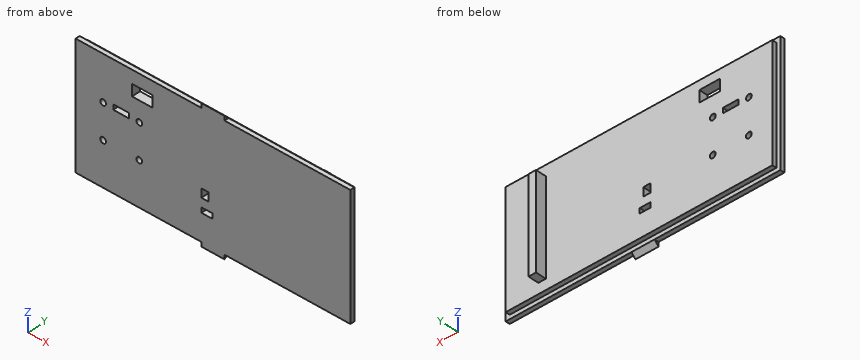
```python
from build123d import *

# Parameters (mm, degrees)
SKETCH2_W               = 190
SKETCH2_H               = 85
BOSS_EXTRUDE1_DEPTH     = 3
SKETCH6_W               = 184.4
SKETCH6_H               = 79.4
BOSS_EXTRUDE4_DEPTH     = 3
SKETCH8_W               = 16
SKETCH8_H               = 3
BOSS_EXTRUDE5_DEPTH     = 3
CHAMFER2_SIZE           = 3
CUT_EXTRUDE1_DEPTH      = 210.475535564
CUT_EXTRUDE1_DEPTH_BACK = 210.475535564
SKETCH10_W              = 7.5
SKETCH10_H              = 3.5
SKETCH11_W              = 5
SKETCH11_H              = 6
CUT_EXTRUDE2_DEPTH      = 210.475535564
SKETCH12_R              = 2
SKETCH12_W              = 11
SKETCH12_H              = 3.5
CUT_EXTRUDE3_DEPTH      = 210.475535564
SKETCH13_W              = 14.2
SKETCH13_H              = 8
CUT_EXTRUDE4_DEPTH      = 210.475535564
SKETCH14_W              = 5.173747918
SKETCH14_H              = 65
BOSS_EXTRUDE6_DEPTH     = 7.3


with BuildPart() as part:
    # Sketch2 → Boss-Extrude1 (new body)
    with BuildSketch(Plane(origin=(0, 0, 0), x_dir=(1, 0, 0), z_dir=(0, 1, 0))):
        with Locations((-95, 42.5)):
            Rectangle(SKETCH2_W, SKETCH2_H)
    extrude(amount=BOSS_EXTRUDE1_DEPTH)

    # Sketch6 → Boss-Extrude4 (add)
    with BuildSketch(Plane(origin=(0, 3, 0), x_dir=(1, 0, 0), z_dir=(0, 1, 0))):
        with Locations((-95, 42.5)):
            Rectangle(SKETCH6_W, SKETCH6_H)
    extrude(amount=BOSS_EXTRUDE4_DEPTH)

    # Sketch8 → Boss-Extrude5 (add)
    with BuildSketch(Plane(origin=(0, 3, 0), x_dir=(1, 0, 0), z_dir=(0, 1, 0))):
        with Locations((-95, -1.5)):
            Rectangle(SKETCH8_W, SKETCH8_H)
        with Locations((-95, 86.5)):
            Rectangle(SKETCH8_W, SKETCH8_H)
    extrude(amount=-BOSS_EXTRUDE5_DEPTH)

    # Chamfer2
    chamfer2_edges = [part.edges().sort_by_distance(p)[0] for p in [
        (-95, 3, 3),
        (-95, 3, -88),
    ]]
    chamfer(chamfer2_edges, length=CHAMFER2_SIZE - 0.0001)  # a hair under: the kernel refuses the full size

    # Sketch10 → Cut-Extrude1 (cut, two sides: drawn at the far end of the back side and taken through both)
    with BuildSketch(Plane.XZ.offset(-CUT_EXTRUDE1_DEPTH_BACK)):
        with Locations((-99.25, -64.75)):
            Rectangle(SKETCH10_W, SKETCH10_H)
    extrude(amount=CUT_EXTRUDE1_DEPTH + CUT_EXTRUDE1_DEPTH_BACK, mode=Mode.SUBTRACT)

    # Sketch11 → Cut-Extrude2 (cut, through all)
    with BuildSketch(Plane.XZ):
        with Locations((-100.5, -54)):
            Rectangle(SKETCH11_W, SKETCH11_H)
    extrude(amount=-CUT_EXTRUDE2_DEPTH, mode=Mode.SUBTRACT)

    # Sketch12 → Cut-Extrude3 (cut, through all)
    with BuildSketch(Plane.XZ):
        with Locations(Location((-171, -54.875455527, 0), (0, 0, 270))):
            Circle(SKETCH12_R)
        with Locations(Location((-171, -30.875455527, 0), (0, 0, 270))):
            Circle(SKETCH12_R)
        with Locations(Location((-146, -54.875455527, 0), (0, 0, 90))):
            Circle(SKETCH12_R)
        with Locations(Location((-146, -30.875455527, 0), (0, 0, 90))):
            Circle(SKETCH12_R)
        with Locations((-158.5, -30.25)):
            Rectangle(SKETCH12_W, SKETCH12_H)
    extrude(amount=-CUT_EXTRUDE3_DEPTH, mode=Mode.SUBTRACT)

    # Sketch13 → Cut-Extrude4 (cut, through all)
    with BuildSketch(Plane.XZ):
        with Locations((-143.9, -13)):
            Rectangle(SKETCH13_W, SKETCH13_H)
    extrude(amount=-CUT_EXTRUDE4_DEPTH, mode=Mode.SUBTRACT)

    # Sketch14 → Boss-Extrude6 (add)
    with BuildSketch(Plane(origin=(0, 6, 0), x_dir=(1, 0, 0), z_dir=(0, 1, 0))):
        with Locations((-27.918538548, 42.5)):
            Rectangle(SKETCH14_W, SKETCH14_H)
    extrude(amount=BOSS_EXTRUDE6_DEPTH)


solid = part.part
```
Geometry check sheet. Reference: the model listing, model coordinates, mm. Coordinates: 2 decimals unless noted, no trailing zeros. Loops run counter-clockwise (first coordinate to the right, second up) from the corner with the lowest first, then second, coordinate; pieces in that order, holes last. Notation, with made-up numbers: (44.25, 23.5) -> (77.25, 23.5) arc R19 cw to (77.25, 36.5) -> close; hole circle Ø1 at (55, 14.25). An arc over 180 degrees is marked (long way). Put each result on its own line as item: value.
1) Thickness scan on line 1 (Z direction, x = -146, y = 1.8); line 2 (X direction, y = 3.25, z = -12); line 3 (Z direction, x = -146, y = 3.2). Record the ranges inside material, lowest first.
Result set:
line 1: z = -85 to -56.88, -52.88 to -32.88, -28.88 to -17, -9 to 0
line 2: x = -187.2 to -151, -136.8 to -2.8
line 3: z = -82.2 to -56.88, -52.88 to -32.88, -28.88 to -17, -9 to -2.8
2) Cross-section at B-B on z = -43.5. Record the boundary of the cut face in (x, y).
Result set:
outline: (-190, 0) -> (0, 0) -> (0, 3) -> (-2.8, 3) -> (-2.8, 6) -> (-25.33, 6) -> (-25.33, 13.3) -> (-30.51, 13.3) -> (-30.51, 6) -> (-187.2, 6) -> (-187.2, 3) -> (-190, 3) -> close
3) Cross-section at C-C on x = -56. Record the boundary of the cut face in (y, z), plus the area to 3 significant figures.
Result set:
outline: (0, -85) -> (3, -85) -> (3, -82.2) -> (6, -82.2) -> (6, -2.8) -> (3, -2.8) -> (3, 0) -> (0, 0) -> close
area: 493 mm^2
4) Gauge pin test, flat ends, axial feed: pin 1 Ø1.5 at (x, y) = (-113, 4) entering from -Z; pin 2 Ø5 at (x, y) = (-164.5, 1.5) entering from +Z; pin 3 Ø3.5 at (x, y) = (-149.5, 2) entering from -Z; pin 4 Ø1.8 at (y, z) = (2.5, -31) entering from +X. Record the tip position at first contact, or that the pin passes through.
Result set:
pin 1: stops at z = -82.2
pin 2: stops at z = 0
pin 3: stops at z = -85
pin 4: stops at x = 0
5) Cross-section at A-A on x = -158. Record the boundary of the cut face in (y, z), plus the area to 3 significant figures.
Result set:
outline: (0, -85) -> (3, -85) -> (3, -82.2) -> (6, -82.2) -> (6, -32) -> (0, -32) -> close; (0, -28.5) -> (6, -28.5) -> (6, -2.8) -> (3, -2.8) -> (3, 0) -> (0, 0) -> close
area: 472 mm^2
